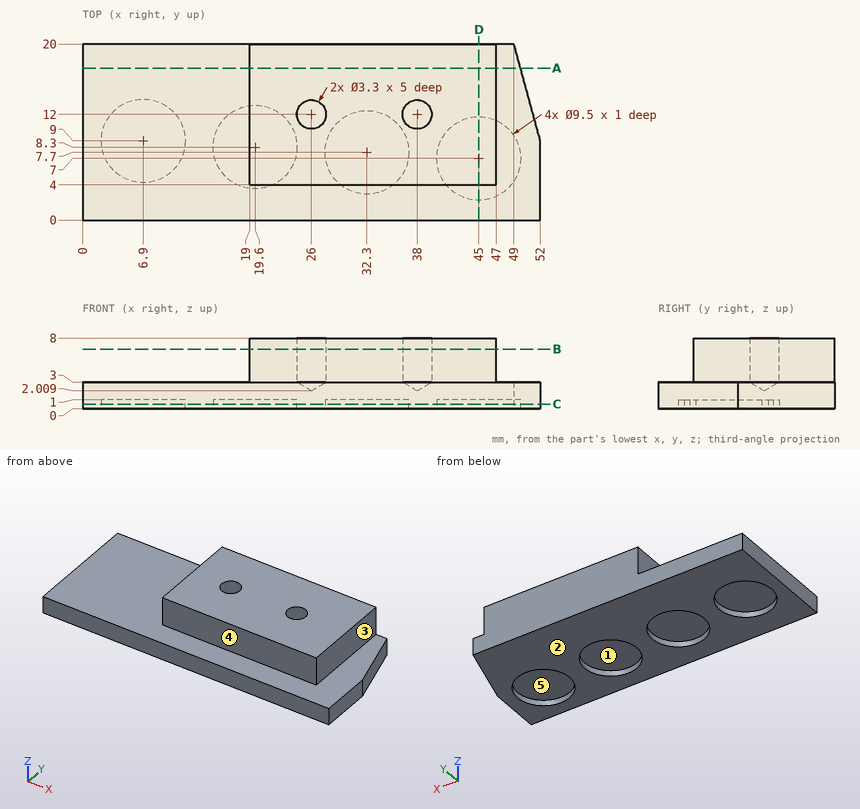
Verification items for this drawing (mm, ordinates from the low corner). A direction names the side the tool comes from. Coordinates: 2 decimals unless noted, no trailing zeros. Write each loop counter-clockwise with the first axis right and the second up, starting at its lowest first coordinate (ties: lowest second). Pieces come first, ordered by that corner, then holes. Notation, with made-up numbers: M -14,85.5 L 21,85.5 A6 ccw 21,92.5 Z; hole C 4.5,10 d11. An arc over 180 degrees is marked long. Use one line per item in the form item = value. Start each with the question number.
1) Section check C-C on z = 0.5. Enter the section's corners in (x, y).
2) Section check A-A on y = 17.25. Enter the section's corners in (x, z), and give its area (3 significant figures).
3) Thickness scan on probe 1 along X at (y, z) = (12, 4.4); probe 2 along Y at (x, z) = (6.9, 0.75); probe 3 along Y at (x, z) = (45, 0.65). Record the ranges inside material, lowest first. Write a range as from..to.
4) Release check for a two-part mould opening along Y. For the marked faces 3, 4 and 5 record: pulls with the +Y half, pulls with the -Y half, needs draft (parallel to the pull), parting line crosses it, or undercut.
5) Section check B-B on z = 6.75. Enter the section's corners in (x, y).
6) Go/stop test with flat-tipped pins: pin 1 Ø1.5 at (y, z) = (14, 6.5) entering from +X; pin 2 Ø8.5 at (x, y) = (6.9, 9) entering from -Z; pin 3 Ø3 at (x, y) = (26, 12) entering from +Z. Record where each tip stops, or that it passes through.
7) Set-up check for the marked faces 1 and 2: record each of +Z, -Z, +X, -X, +Y, -Y from which the full face is reachable in a straight line by a thin tool's end or side.
8) Section check D-D on x = 45. Enter the section's corners in (y, z), and give its area (4 significant figures).
Responses:
q1.outline = M 0,0 L 52,0 L 52,9 L 49,20 L 0,20 Z; hole C 6.9,9 d9.5; hole C 19.6,8.3 d9.5; hole C 32.3,7.7 d9.5; hole C 45,7 d9.5
q2.outline = M 0,0 L 49.75,0 L 49.75,3 L 47,3 L 47,8 L 19,8 L 19,3 L 0,3 Z
q2.area = 289 mm2
q3.probe_1 = 19..24.35, 27.65..36.35, 39.65..47
q3.probe_2 = 0..4.25, 13.75..20
q3.probe_3 = 0..2.25, 11.75..20
q4.face_3 = needs draft
q4.face_4 = pulls with the -Y half
q4.face_5 = undercut
q5.outline = M 19,4 L 47,4 L 47,20 L 19,20 Z; hole C 26,12 d3.3; hole C 38,12 d3.3
q6.pin_1 = 47
q6.pin_2 = 1
q6.pin_3 = 2.91
q7.face_1 = -Z
q7.face_2 = -Z, +X, -X, +Y, -Y
q8.outline = M 0,0 L 2.25,0 L 2.25,1 L 11.75,1 L 11.75,0 L 20,0 L 20,8 L 4,8 L 4,3 L 0,3 Z
q8.area = 130.5 mm2
